Design review of the part built by this model. Coordinates are the model's own, in mm. Face numbers are marked on the shaded views. A direction names the side the tool comes from. Coordinates: 2 decimals unless noted, no trailing zeros. Loops run counter-clockwise (first coordinate to the right, second up) from the corner with the lowest first, then second, coordinate; pieces in that order, holes last. Notation, with made-up numbers: (23.25, 65) -> (38.25, 65) arc R21 ccw to (38.25, 99) -> close; hole circle Ø7 at (56.25, -27.5). An arc over 180 degrees is marked (long way). Answer as a JSON object with one key per item and string values.
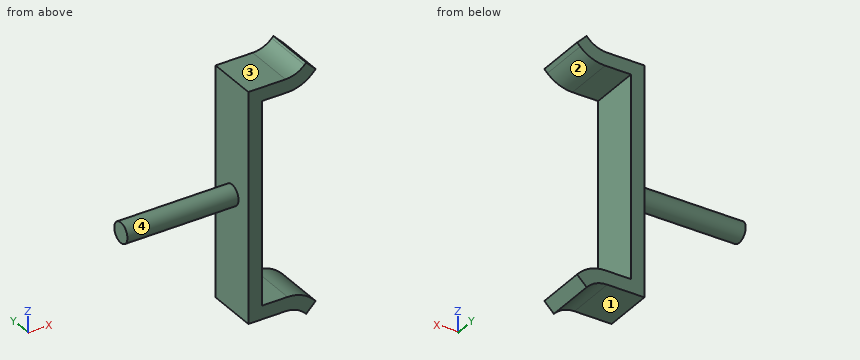
```python
from build123d import *

# Parameters (mm, degrees)
BOSS_EXTRUDE2_DEPTH = 15
SKETCH3_R           = 3
BOSS_EXTRUDE3_DEPTH = 33


with BuildPart() as part:
    # Sketch1 → Boss-Extrude2 (new body)
    with BuildSketch(Plane(origin=(0, 0, 0), x_dir=(1, 0, 0), z_dir=(0, 1, 0))):
        with BuildLine():
            Line((0, 34), (0, 0))
            Line((0, 0), (4, 0))
            Line((4, 0), (4, 30))
            Line((4, 30), (11.650757595, 30))
            ThreePointArc((11.650757595, 30), (15.668933635, 30.799264909), (19.075378798, 33.075378798))
            Line((19.075378798, 33.075378798), (20, 34))
            Line((20, 34), (17.171572875, 36.828427125))
            Line((17.171572875, 36.828427125), (16.686291501, 36.343145751))
            ThreePointArc((16.686291501, 36.343145751), (14.09090471, 34.60896374), (11.029437252, 34))
            Line((11.029437252, 34), (0, 34))
        make_face()
        with BuildLine():
            Line((0, 0), (0, -34))
            Line((0, -34), (11.029437252, -34))
            ThreePointArc((11.029437252, -34), (14.09090471, -34.60896374), (16.686291501, -36.343145751))
            Line((16.686291501, -36.343145751), (17.171572875, -36.828427125))
            Line((17.171572875, -36.828427125), (20, -34))
            Line((20, -34), (19.075378798, -33.075378798))
            ThreePointArc((19.075378798, -33.075378798), (15.668933635, -30.799264909), (11.650757595, -30))
            Line((11.650757595, -30), (4, -30))
            Line((4, -30), (4, 0))
            Line((4, 0), (0, 0))
        make_face()
    extrude(amount=BOSS_EXTRUDE2_DEPTH)

    # Sketch3 → Boss-Extrude3 (add)
    with BuildSketch(Plane.ZY):
        with Locations((0, 7.5)):
            Circle(SKETCH3_R)
    extrude(amount=BOSS_EXTRUDE3_DEPTH)


solid = part.part
```
1) Add section D-D, the plane x = 15. Give the boundary of the cut face in (y, z).
Completed:
{"outline": "(0, -35.05) -> (15, -35.05) -> (15, -30.55) -> (0, -30.55) -> close; (0, 30.55) -> (15, 30.55) -> (15, 35.05) -> (0, 35.05) -> close"}
2) Clearance check with flat-ended pins moving along their axes: pin 1 Ø6 at (y, z) = (3, 28) entering from -X; pin 2 Ø9 at (x, y) = (5, 10) entering from -Z; pin 3 Ø1.5 at (x, z) = (-25.5, 2.5) entering from +Y. State where each tip first meets the part, or that it passes through.
Completed:
{"pin 1": "x = 0", "pin 2": "z = -34", "pin 3": "y = 9.94"}
3) Add section A-A, the plane x = 9. Give the boundary of the cut face in (y, z).
Completed:
{"outline": "(0, -34) -> (15, -34) -> (15, -30) -> (0, -30) -> close; (0, 30) -> (15, 30) -> (15, 34) -> (0, 34) -> close"}
4) Add section C-C, the plane z = 0. Give the boundary of the cut face in (x, y), and give its area (3 significant figures).
Completed:
{"outline": "(-33, 4.5) -> (0, 4.5) -> (0, 0) -> (4, 0) -> (4, 15) -> (0, 15) -> (0, 10.5) -> (-33, 10.5) -> close", "area": "258 mm²"}
5) Add section B-B, the plane y = 7.5. Give the boundary of the cut face in (x, z).
Completed:
{"outline": "(-33, -3) -> (0, -3) -> (0, -34) -> (11.03, -34) arc R8 cw to (16.69, -36.34) -> (17.17, -36.83) -> (20, -34) -> (19.08, -33.08) arc R10.5 ccw to (11.65, -30) -> (4, -30) -> (4, 30) -> (11.65, 30) arc R10.5 ccw to (19.08, 33.08) -> (20, 34) -> (17.17, 36.83) -> (16.69, 36.34) arc R8 cw to (11.03, 34) -> (0, 34) -> (0, 3) -> (-33, 3) -> close"}
6) For the marked faces 1, 2, 3 and 4, list the 3-axis set-ups (+Z, -Z, +X, -X, +Y, -Y) from which the entire face can be reached by the end or side of a thin tool; tool diameter is ignored.
Completed:
{"face 1": "-Z, -X, +Y, -Y", "face 2": "+X, +Y, -Y", "face 3": "+Z, -X, +Y, -Y", "face 4": "-X"}
7) Wall thickness on probe 1 along Z at (x, y) = (11.5, 10); probe 2 along X at (y, z) = (2.25, 2); probe 3 along Z at (x, y) = (2.5, 13.5): over which ranges is each line inside the solid? List them lowest first.
Completed:
{"probe 1": "-34.01 to -30, 30 to 34.01", "probe 2": "0 to 4", "probe 3": "-34 to 34"}
